Geometry check sheet. Reference: drawing and pictorial views, mm from the part's lowest x, y, z. A direction names the side the tool comes from. Round coordinates to 2 decimals unless told otherwise and drop trailing zeros. Write each loop counter-clockwise with the first axis right and the second up, starting at its lowest first coordinate (ties: lowest second). Pieces come first, ordered by that corner, then holes. Notation, with made-up numbers: (2.25, 58.5) -> (9.25, 58.5) arc R18 cw to (9.25, 77.5) -> close; hole circle Ø9 at (30.25, 48.25). An arc over 180 degrees is marked (long way). Write item = value, one per line.
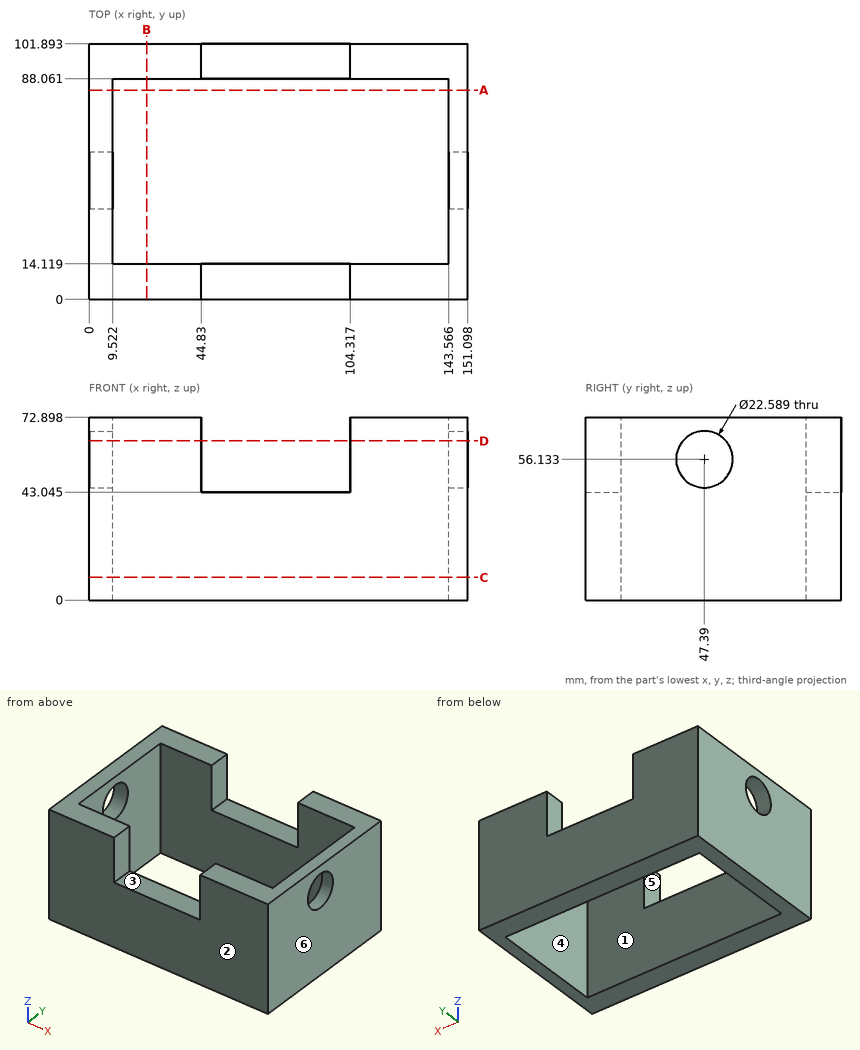
(1) Sectioned sample at A-A on y = 83.5. Enter the section's corners in (x, z), then the cut area to 3 significant figures.
Worked answers:
outline = (0, 0) -> (9.52, 0) -> (9.52, 72.9) -> (0, 72.9) -> close; (143.57, 0) -> (151.1, 0) -> (151.1, 72.9) -> (143.57, 72.9) -> close
area = 1,240 mm²
(2) Access from +Z, -Z, +X, -X, +Y, -Y to the whole of each face (thin tool, end or side, straight path). Record for the marked faces 4, 5 and 6.
Worked answers:
face_4 = +Z, -Z
face_5 = +Z, +Y, -Y
face_6 = +Z, -Z, +X, +Y, -Y
(3) Sectioned sample at D-D on z = 63.5. Enter the section's corners in (x, y), then the cut area to 3 significant figures.
Worked answers:
outline = (0, 0) -> (44.83, 0) -> (44.83, 14.12) -> (9.52, 14.12) -> (9.52, 38.83) -> (0, 38.83) -> close; (0, 55.95) -> (9.52, 55.95) -> (9.52, 88.06) -> (44.83, 88.06) -> (44.83, 101.89) -> (0, 101.89) -> close; (104.32, 0) -> (151.1, 0) -> (151.1, 38.83) -> (143.57, 38.83) -> (143.57, 14.12) -> (104.32, 14.12) -> close; (104.32, 88.06) -> (143.57, 88.06) -> (143.57, 55.95) -> (151.1, 55.95) -> (151.1, 101.89) -> (104.32, 101.89) -> close
area = 3,530 mm²
(4) Go/stop test with flat-tipped pins: P1, Ø18, axis at y = 47.39, z = 56.13, coming from the -X side; P2, Ø15, axis at x = 63, y = 98.5, coming from the +Z side (1 decimal). Record where each tip stops, or that it passes through.
Worked answers:
P1 = through
P2 = 43
(5) Material ranges on L1, parallel to X at y = 19.5, z = 56; L2, parallel to Y at x = 44.5, z = 22; L3, parallel to X at y = 94, z = 60, recorded low to high. Write a range as [from, to].
Worked answers:
L1 = [0, 9.52], [143.57, 151.1]
L2 = [0, 14.12], [88.06, 101.89]
L3 = [0, 44.83], [104.32, 151.1]
(6) Sectioned sample at B-B on x = 23. Enter the section's corners in (y, z).
Worked answers:
outline = (0, 0) -> (14.12, 0) -> (14.12, 72.9) -> (0, 72.9) -> close; (88.06, 0) -> (101.89, 0) -> (101.89, 72.9) -> (88.06, 72.9) -> close
(7) Sectioned sample at C-C on z = 9. Enter the section's corners in (x, y).
Worked answers:
outline = (0, 0) -> (151.1, 0) -> (151.1, 101.89) -> (0, 101.89) -> close; hole (9.52, 14.12) -> (143.57, 14.12) -> (143.57, 88.06) -> (9.52, 88.06) -> close
(8) Release check for a two-part mould opening along Y. For the marked faces 1, 2 and 3 record: pulls with the +Y half, pulls with the -Y half, needs draft (parallel to the pull), parting line crosses it, or undercut.
Worked answers:
face_1 = undercut
face_2 = pulls with the -Y half
face_3 = needs draft
